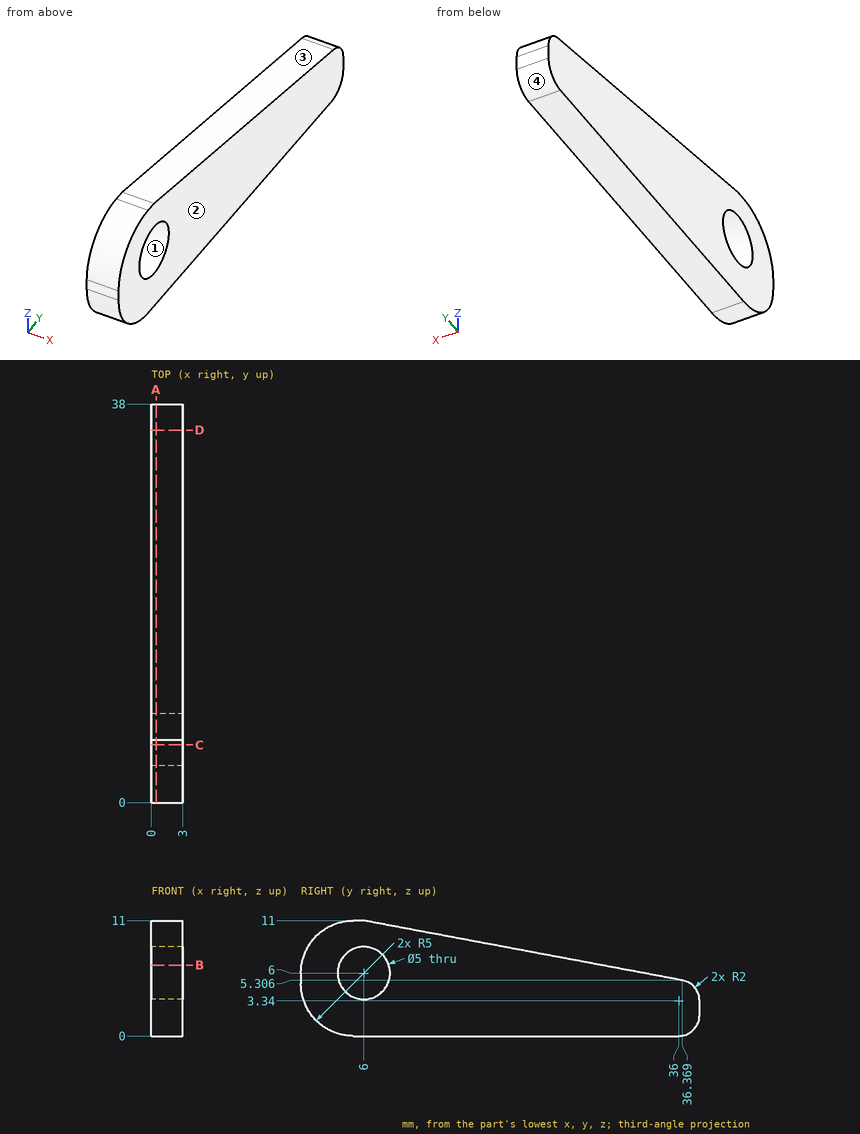
The drawing under review shows one solid part. Ordinate dimensions are in mm from its lowest x, y, z. Round coordinates to 2 decimals unless told otherwise and drop trailing zeros. Write each loop counter-clockwise with the first axis right and the second up, starting at its lowest first coordinate (ties: lowest second). Pieces come first, ordered by that corner, then holes. Notation, with made-up numbers: M 6.5,36 L 29.5,36 A3 cw 29.5,40 Z; hole C 32,-1 d1. An arc over 180 degrees is marked long. One line per item, written item: value. Start each with the question number.
(1) We need section B-B (z = 6.75). Give the boundary of the cut face in (x, y) (1 decimal).
(2) The part is to be moulded in two halves that separate along Z. For the marked faces 1, 2, 3 and 4, say which applies: released by +Z, released by -Z, zero draft, split by the parting line, or undercut.
(3) We need section C-C (y = 5.5). Give the boundary of the cut face in (x, z).
(4) Insertion check: pin 1 (6 mm diameter, centred on y = 6, z = 6, fed in from +X). The pin has a flat end and moves straight along its axis. Give the tip position at first contact, or say it passes through.
(5) We need section A-A (x = 0.45). Give the boundary of the cut face in (y, z).
(6) Wall thickness on line 1 (Z direction, x = 0.9, y = 6); line 2 (Y direction, x = 0.35, z = 3.25) (1 decimal); line 3 (Z direction, x = 2.25, y = 18.5): over which ranges is each line inside the solid? List them lowest first.
(7) We need section D-D (y = 35.5). Give the boundary of the cut face in (x, z).
Result:
1. outline: M 0,0.1 L 3,0.1 L 3,3.6 L 0,3.6 Z; M 0,8.4 L 3,8.4 L 3,28.7 L 0,28.7 Z
2. face 1: undercut
2. face 2: zero draft
2. face 3: released by +Z
2. face 4: released by -Z
3. outline: M 0,0 L 3,0 L 3,3.55 L 0,3.55 Z; M 0,8.45 L 3,8.45 L 3,11 L 0,11 Z
4. pin 1: x = 3
5. outline: M 0,5 A5 ccw 5,0 L 36,0 A2 ccw 38,2 L 38,3.34 A2 ccw 36.37,5.31 L 6,11 L 5,11 A5 ccw 0,6 Z; hole C 6,6 d5
6. line 1: 0 to 3.5, 8.5 to 11
6. line 2: 0.3 to 38
6. line 3: 0 to 8.66
7. outline: M 0,0 L 3,0 L 3,5.47 L 0,5.47 Z
